The listing builds one solid part. Answer for the finished solid, in the listing's coordinates (mm). A direction names the side the tool comes from. Give positions to 0.01 mm unless a question says otherwise; leave off trailing zeros. Loops run counter-clockwise (first coordinate to the right, second up) from the corner with the lowest first, then second, coordinate; pieces in that order, holes last. Notation, with made-up numbers: M -22,-18 L -16,-18 A16 ccw -16,-6 Z; hole C 63,-27 d4. An arc over 180 degrees is marked long. One line per item, written item: value. Start each with the question number.
Q1. Flat-ended cylindrical pins translate along their axes: pin 1 (8 mm diameter, centred on x = -1.5, y = -3, fed in from -Z); pin 2 (1.5 mm diameter, centred on y = -1, z = 3, fed in from -X); pin 3 (3.5 mm diameter, centred on y = -2, z = -4, fed in from +X); pin 4 (0.6 mm diameter, centred on x = 9.5, z = 9, fed in from -Y). Find the tip coordinate at first contact, or state that the pin passes through.
Q2. A cutting plane is placed at D-D, the plane z = -5.75. Determine the outline of the cut face in (x, y).
Q3. Consider L1, parallel to Y at x = -10.2, z = 0; L2, parallel to Z at x = -2.25, y = -0.25; L3, parallel to Z at x = 3, y = -2. Determine where each line is inside the solid, lowest interval first.
Q4. The mould has two halves that part along X. Classify faces 1 (the cylindrical face through (9.225, 0.01, 9.387)), 2 (the cylindrical face through (0.81, -7.05, -8.24)), 3 (the cylindrical face through (-9.419, -6.936, -0.106)), 4 (the cylindrical face through (9.225, 0.01, -9.387)): +X half, -X half, draft (parallel to the pull), parting line (faces both ways), or undercut.
Q5. A cutting plane is placed at B-B, the plane z = 0.5. Determine the outline of the cut face in (x, y), and give its area (3 significant figures).
Q6. For faces 5 (the flat face through (-0.369, 7.405, 4.289)), 6 (the flat face through (5, 7.25, 0)), 7 (the cylindrical face through (-10.5, 0.1, -3)), determine the directions among +Z, -Z, +X, -X, +Y, -Y from which every point of the face is accessible in a straight line to the end or side of a thin tool.
Q7. A cutting plane is placed at C-C, the plane x = -6.25. Determine the outline of the cut face in (y, z).
Q8. A cutting plane is placed at A-A, the plane x = 0.75. Determine the outline of the cut face in (y, z), and give its area (3 significant figures).
from build123d import *

# Parameters (mm, degrees)
BOSS_EXTRUDE1_DEPTH       = 10
SKETCH2_R                 = 3
BOSS_EXTRUDE3_DEPTH       = 1
FILLET2_R                 = 1.35
SHELL6_T                  = -0.25
SHELL6_THICKNESS_2_FACE_R = 2.75
SHELL6_THICKNESS_2_DEPTH  = 1
SKETCH3_R                 = 1
CUT_EXTRUDE2_DEPTH        = 25.438698861
CUT_EXTRUDE6_DEPTH        = 10
CUT_EXTRUDE9_DEPTH        = 17.650825865
CUT_EXTRUDE9_DEPTH_BACK   = 17.650825865
BOSS_EXTRUDE4_DEPTH       = 0.75
FILLET3_R                 = 0.4
FILLET3_OF_MIRROR2_R      = 0.4


with BuildPart() as part:
    # Sketch1 → Boss-Extrude1 (new, symmetric)
    with BuildSketch(Plane(origin=(0, 0, 0), x_dir=(0, 0, -1), z_dir=(1, 0, 0))):
        with BuildLine():
            Line((-8.540496218, -7.5), (8.540496218, -7.5))
            ThreePointArc((8.540496218, -7.5), (10, 0), (8.540496218, 7.5))
            Line((8.540496218, 7.5), (-8.540496218, 7.5))
            ThreePointArc((-8.540496218, 7.5), (-10, 0), (-8.540496218, -7.5))
        make_face()
    extrude(amount=BOSS_EXTRUDE1_DEPTH, both=True)

    # Sketch2 → Boss-Extrude3 (add)
    with BuildSketch(Plane.ZY.offset(10)):
        Circle(SKETCH2_R)
    extrude(amount=BOSS_EXTRUDE3_DEPTH)

    # Fillet2
    fillet2_edges = [part.edges().sort_by_distance(p)[0] for p in [
        (-10, -7.5, 0),
        (-10, 0, 10),
        (-10, 7.5, 0),
        (-10, 0, -10),
        (0, -7.5, -8.540496218),
        (0, -7.5, 8.540496218),
        (0, 7.5, 8.540496218),
        (0, 7.5, -8.540496218),
    ]]
    fillet(fillet2_edges, radius=FILLET2_R)

    # Shell6
    shell6_openings = [part.faces().sort_by_distance(p)[0] for p in [
        (10, 0, 0),
    ]]
    offset(amount=SHELL6_T, openings=shell6_openings, kind=Kind.INTERSECTION)

    # Shell6 thickness 2 face (on inner face of the shell) → Shell6 thickness 2 (add)
    with BuildSketch(Plane(origin=(-10.75, 0, 0), x_dir=(0, 0, -1), z_dir=(-1, 0, 0))):
        Circle(SHELL6_THICKNESS_2_FACE_R)
    extrude(amount=-SHELL6_THICKNESS_2_DEPTH)

    # Sketch3 → Cut-Extrude2 (cut, through all)
    with BuildSketch(Plane.ZY.offset(11)):
        Circle(SKETCH3_R)
    extrude(amount=-CUT_EXTRUDE2_DEPTH, mode=Mode.SUBTRACT)

    # Sketch8 → Cut-Extrude6 (cut)
    with BuildSketch(Plane(origin=(0, 1.317628396, 9.375413194), x_dir=(-1, 0, 0), z_dir=(0, -0.13917310096005872, -0.9902680687415713))):
        Polygon((3.5, 6.735543413), (3.5, 7.235543413), (-3.5, 7.235543413), (-3.5, 7.035543413), (-2.675756774, 6.735543413), align=None)
    cut_extrude6 = extrude(amount=CUT_EXTRUDE6_DEPTH, mode=Mode.SUBTRACT)

    # Mirror1: Cut-Extrude6 across plane
    add(cut_extrude6.mirror(Plane.XY), mode=Mode.SUBTRACT)

    # Sketch9 → Cut-Extrude9 (cut, two sides: drawn at the far end of the back side and taken through both)
    with BuildSketch(Plane.XY.offset(-CUT_EXTRUDE9_DEPTH_BACK)):
        with BuildLine():
            Line((10, 1.975), (9, 1.975))
            ThreePointArc((9, 1.975), (8.646446609, 1.828553391), (8.5, 1.475))
            Line((8.5, 1.475), (8.5, -1.475))
            ThreePointArc((8.5, -1.475), (8.646446609, -1.828553391), (9, -1.975))
            Line((9, -1.975), (10, -1.975))
            Line((10, -1.975), (10, 1.975))
        make_face()
    extrude(amount=CUT_EXTRUDE9_DEPTH + CUT_EXTRUDE9_DEPTH_BACK, mode=Mode.SUBTRACT)

    # Sketch10 → Boss-Extrude4 (add, symmetric)
    with BuildSketch(Plane(origin=(0, 0, 0), x_dir=(1, 0, 0), z_dir=(0, 1, 0))):
        with BuildLine():
            Line((9.787254425, 8.770946884), (10, 8.902245476))
            ThreePointArc((10, 8.902245476), (9.357045131, 9.600790595), (8.5, 10.009238743))
            Line((8.5, 10.009238743), (8.5, 9.75))
            ThreePointArc((8.5, 9.75), (9.234633876, 9.380128574), (9.787254425, 8.770946884))
        make_face()
    boss_extrude4 = extrude(amount=BOSS_EXTRUDE4_DEPTH, both=True)

    # Fillet3
    # the kernel refuses this fillet: 0.4 mm, written as the material it takes off along each edge
    with BuildSketch(Plane(origin=(10, -1.816179824, -8.902245476), x_dir=(-0.5958644657963694, 0, -0.8030850131842876), z_dir=(0, 1, 0))) as fillet3_piece_1:
        with BuildLine():
            CenterArc((0.392354175, 0.398542317), FILLET3_R, 201.939875172, 72.953078249)
            Line((0.021323596, 0.249088948), (0.013902985, 0.246099881))
            ThreePointArc((0.013902985, 0.246099881), (0.002690952, 0.125226829), (-0.007970846, 0.000682355))
            Line((-0.007970846, 0.000682355), (-0.000682355, -0.007970846))
            ThreePointArc((-0.000682355, -0.007970846), (0.213235965, -0.017110516), (0.427154285, -0.007970846))
            Line((0.427154285, -0.007970846), (0.42647193, 0))
        make_face()
    extrude(amount=3.632359649, mode=Mode.SUBTRACT)

    # Mirror2: Boss-Extrude4 across plane
    add(boss_extrude4.mirror(Plane.XY))

    # Fillet3 of Mirror2
    # the kernel refuses this fillet: 0.4 mm, written as the material it takes off along each edge
    with BuildSketch(Plane(origin=(10, -1.816179824, 8.902245476), x_dir=(-0.5958644657963694, 0, 0.8030850131842876), z_dir=(0, 1, 0))) as fillet3_of_mirror2_piece_1:
        with BuildLine():
            CenterArc((0.392354175, -0.398542317), FILLET3_OF_MIRROR2_R, 85.10704658, 72.953078249)
            Line((0.021323596, -0.249088948), (0.013902985, -0.246099881))
            ThreePointArc((0.013902985, -0.246099881), (0.002690952, -0.125226829), (-0.007970846, -0.000682355))
            Line((-0.007970846, -0.000682355), (-0.000682355, 0.007970846))
            ThreePointArc((-0.000682355, 0.007970846), (0.213235965, 0.017110516), (0.427154285, 0.007970846))
            Line((0.427154285, 0.007970846), (0.42647193, 0))
        make_face()
    extrude(amount=3.632359649, mode=Mode.SUBTRACT)


solid = part.part
Answer block:
1. pin 1: z = -10
1. pin 2: x = -11
1. pin 3: x = -9.75
1. pin 4: y = -6.94
2. outline: M -10,-6.15 A1.35 ccw -8.65,-7.5 L 10,-7.5 L 10,-7.25 L -8.65,-7.25 A1.1 cw -9.75,-6.15 L -9.75,6.15 A1.1 cw -8.65,7.25 L 10,7.25 L 10,7.5 L -8.65,7.5 A1.35 ccw -10,6.15 Z
3. L1: -3 to -1, 1 to 3
3. L2: -10 to -9.75, 9.75 to 10
3. L3: -9.9 to -9.65, 9.65 to 9.9
4. face 1: undercut
4. face 2: draft
4. face 3: +X half
4. face 4: undercut
5. outline: M -11,-2.96 L -10,-2.96 L -10,-6.15 A1.35 ccw -8.65,-7.5 L 10,-7.5 L 10,-7.25 L -8.65,-7.25 A1.1 cw -9.75,-6.15 L -9.75,-0.87 L -11,-0.87 Z; M -11,0.87 L -9.75,0.87 L -9.75,6.15 A1.1 cw -8.65,7.25 L -3.5,7.25 L -3.5,7.38 L 3.5,7.38 L 3.5,7.25 L 10,7.25 L 10,7.5 L -8.65,7.5 A1.35 ccw -10,6.15 L -10,2.96 L -11,2.96 Z
5. area: 16.2 mm^2
6. face 5: +Y
6. face 6: +X
6. face 7: -X
7. outline: M -7.5,-7.61 A1.35 ccw -6.6,-8.88 A20 ccw 6.6,-8.88 A1.35 ccw 7.5,-7.61 L 7.5,7.61 A1.35 ccw 6.6,8.88 A20 ccw -6.6,8.88 A1.35 ccw -7.5,7.61 Z; hole M -7.25,-7.61 A1.1 ccw -6.51,-8.65 A19.75 ccw 6.51,-8.65 A1.1 ccw 7.25,-7.61 L 7.25,7.61 A1.1 ccw 6.51,8.65 A19.75 ccw -6.51,8.65 A1.1 ccw -7.25,7.61 Z
8. outline: M -7.5,-7.61 A1.35 ccw -6.6,-8.88 A20 ccw 6.6,-8.88 A1.35 ccw 7.5,-7.61 L 7.5,-4.97 L 7.25,-3.19 L 7.25,-7.61 A1.1 cw 6.51,-8.65 A19.75 cw -6.51,-8.65 A1.1 cw -7.25,-7.61 L -7.25,7.61 A1.1 cw -6.51,8.65 A19.75 cw 6.51,8.65 A1.1 cw 7.25,7.61 L 7.25,3.19 L 7.5,4.97 L 7.5,7.61 A1.35 ccw 6.6,8.88 A20 ccw -6.6,8.88 A1.35 ccw -7.5,7.61 Z; M 7.31,0 L 7.5,-1.38 L 7.5,1.38 Z
8. area: 14.0 mm^2
